Can you work these out from the drawing? Everything is in mm from the part's minimum corner. A direction names the side the tool comes from. Coordinates: 2 decimals unless noted, no trailing zeros. Write each loop counter-clockwise with the first axis right and the second up, starting at its lowest first coordinate (ties: lowest second). Pieces come first, ordered by that corner, then holes. Notation, with made-up numbers: M 86.5,-23.75 L 116.5,-23.75 A17 cw 116.5,-18.75 Z; hole C 82.5,-19.75 d1. An arc over 180 degrees is marked long. Answer as a JSON object with one key per item and string values. Group by question number.
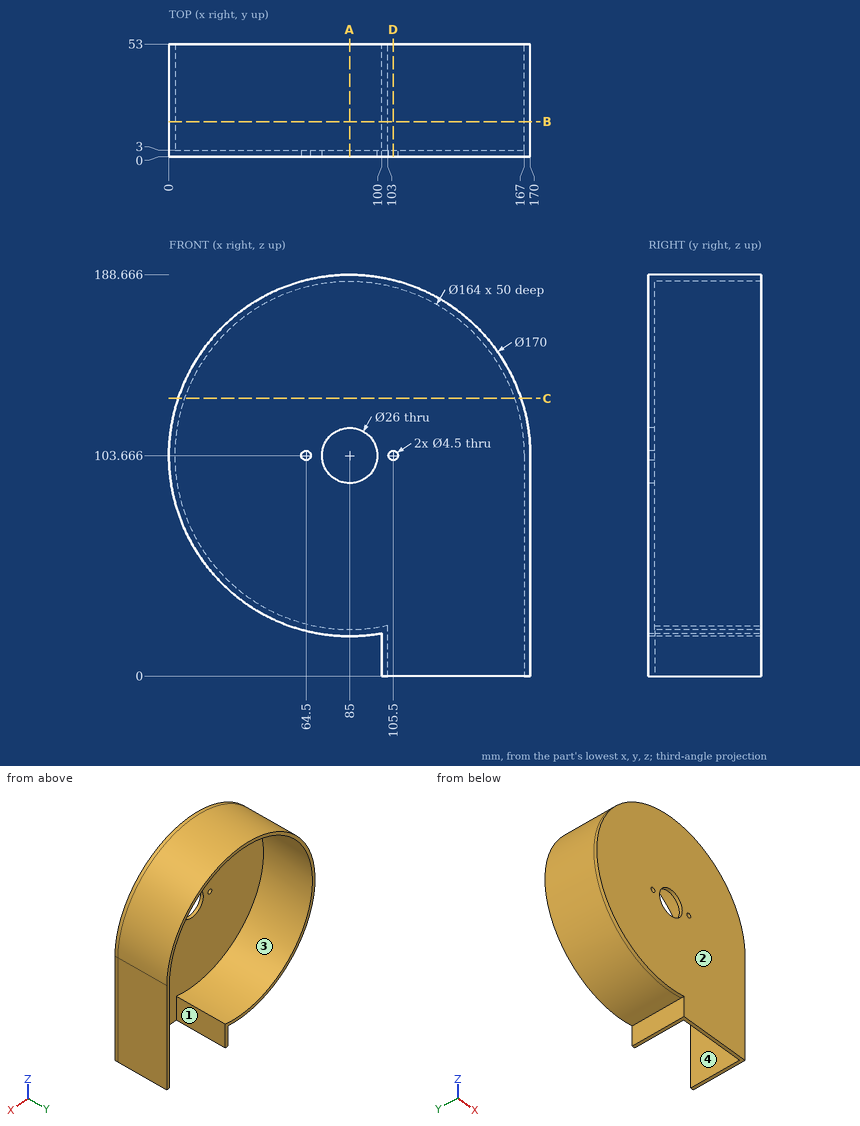
Q1. Please list where these lines run through material, in increasing order: L1, parallel to X at y = 4.5, z = 9; L2, parallel to Z at x = 83.5, y = 17.5; L3, parallel to Z at x = 85, y = 20.
Q2. Will these pins go through, and if not, where does the flat tip stop? pin 1 (6 mm diameter, centred on x = 73.5, y = 14, fed in from -Z); pin 2 (3 mm diameter, centred on x = 67, z = 90, fed in from +Y); pin 3 (1 mm diameter, centred on y = 8.5, z = 162, fed in from -X); pin 4 (15.5 mm diameter, centred on x = 85, z = 103.67, fed in from -Y).
Q3. If we section it at C-C on z = 130.5: List the corners of the cut face in (x, y) for me.
Q4. On a 3-axis mill with a long thin cutter (end or side, diameter ignored), from which of +Z, -Z, +X, -X, +Y, -Y can I reach the whole of each face in a straight line? I mean the marked faces 3 and 4. Say none if no direction works.
Q5. If we section it at B-B on y = 16.5: List the corners of the cut face in (x, z) for me.
Q6. If we section it at A-A on x = 85: List the corners of the cut face in (y, z) for me.
Q7. If we section it at D-D on x = 105.5: List the corners of the cut face in (y, z) for me, and give its area (3 significant figures).
Q8. We'd pull the mould along X, two halves only. Please class the marked faces 1 and 2: pulls with the +X half, pulls with the -X half, needs draft (parallel to the pull), parting line crosses it, or undercut.
Reply:
{
 "1": {"L1": "100 to 103, 167 to 170", "L2": "18.68 to 21.68, 185.65 to 188.65", "L3": "18.67 to 21.67, 185.67 to 188.67"},
 "2": {"pin 1": "z = 19.09", "pin 2": "y = 3", "pin 3": "x = 22.71", "pin 4": "through"},
 "3": {"outline": "M 4.35,0 L 165.65,0 L 165.65,53 L 162.49,53 L 162.49,3 L 7.51,3 L 7.51,53 L 4.35,53 Z"},
 "4": {"face 3": "+Y", "face 4": "-Z, +Y"},
 "5": {"outline": "M 100,0 L 103,0 L 103,23.67 A82 cw long 167,103.67 L 167,0 L 170,0 L 170,103.67 A85 ccw long 100,20 Z"},
 "6": {"outline": "M 0,18.67 L 53,18.67 L 53,21.67 L 3,21.67 L 3,90.67 L 0,90.67 Z; M 0,116.67 L 3,116.67 L 3,185.67 L 53,185.67 L 53,188.67 L 0,188.67 Z"},
 "7": {"outline": "M 0,0 L 3,0 L 3,101.42 L 0,101.42 Z; M 0,105.92 L 3,105.92 L 3,183.06 L 53,183.06 L 53,186.16 L 0,186.16 Z", "area": "700 mm^2"},
 "8": {"face 1": "undercut", "face 2": "needs draft"}
}
